from build123d import *

# Parameters (mm, degrees)
BOSS_EXTRUDE1_DEPTH = 63.5


with BuildPart() as part:
    # Sketch1 → Boss-Extrude1 (new, symmetric)
    with BuildSketch(Plane.XY):
        with BuildLine():
            Line((0, 16.100640303), (0, 50.8))
            Line((0, 50.8), (1.5875, 50.8))
            Line((1.5875, 50.8), (1.5875, 16.758204333))
            ThreePointArc((1.5875, 16.758204333), (2.070864969, 14.328164537), (3.447371939, 12.268076272))
            Line((3.447371939, 12.268076272), (14.592916197, 1.122532015))
            Line((14.592916197, 1.122532015), (13.470384182, 0))
            Line((13.470384182, 0), (1.859871939, 11.610512242))
            ThreePointArc((1.859871939, 11.610512242), (0.483364969, 13.670600507), (0, 16.100640303))
        make_face()
    extrude(amount=BOSS_EXTRUDE1_DEPTH, both=True)


solid = part.part
Verification items for the finished model (mm, model axes). A direction names the side the tool comes from. Give positions to 0.01 mm unless a question says otherwise; leave off trailing zeros. Write each loop counter-clockwise with the first axis right and the second up, starting at its lowest first coordinate (ties: lowest second). Pieces come first, ordered by that corner, then holes. Notation, with made-up numbers: M 39.25,6 L 79.25,6 A34 ccw 79.25,44 Z; hole C 85.25,-10.5 d3. An arc over 180 degrees is marked long. Put each result on its own line as item: value. Start each with the question number.
1. Section check A-A (z = 33). Record the cut outline in (x, y), and give its area (3 significant figures).
2. Scan lines: line 1 along X through (y, z) = (40, 14); line 2 along Y through (x, z) = (6.75, 10.5); line 3 along Y through (x, z) = (3.75, 9). Record each from-to range of solid material in increasing order. Write a range as [from, to].
3. Go/stop test with flat-tipped pins: pin 1 Ø3 at (x, z) = (5.5, -13.5) entering from +Y; pin 2 Ø5 at (y, z) = (16, -37.5) entering from +X; pin 3 Ø2 at (x, z) = (12, -7) entering from +Y. Record where each tip stops, or that it passes through.
4. Section check C-C (x = 11). Record the cut outline in (y, z).
5. Set-up check for faces 1 (the face through (1.588, 34, 1)), 2 (the face through (1, 24, 63.5)): record each of +Z, -Z, +X, -X, +Y, -Y from which the full face is reachable in a straight line by a thin tool's end or side.
6. Section check B-B (y = 24). Record the cut outline in (x, z).
Answer list:
1. outline: M 0,16.1 A6.35 ccw 1.86,11.61 L 13.47,0 L 14.59,1.12 L 3.45,12.27 A6.35 cw 1.59,16.76 L 1.59,50.8 L 0,50.8 Z
1. area: 88.5 mm2
2. line 1: [0, 1.59]
2. line 2: [6.72, 8.97]
2. line 3: [9.72, 11.97]
3. pin 1: y = 11.72
3. pin 2: x = 2.49
3. pin 3: y = 4.72
4. outline: M 2.47,-63.5 L 4.72,-63.5 L 4.72,63.5 L 2.47,63.5 Z
5. face 1: +Z, -Z, +X, +Y
5. face 2: +Z, +X, -X, +Y, -Y
6. outline: M 0,-63.5 L 1.59,-63.5 L 1.59,63.5 L 0,63.5 Z
